from build123d import *

# Parameters (mm, degrees)
F0_W     = 676.275
F0_H     = 650.875
F1_DEPTH = 927.1
F3_DEPTH = 676.275
F4_W     = 473.075
F4_H     = 25.4
F5_DEPTH = 381


with BuildPart() as f1:
    # F0 (on Top) → F1 (new body)
    with BuildSketch(Plane.XY):
        with Locations((2.333625, 72.26744)):
            Rectangle(F0_W, F0_H)
    extrude(amount=F1_DEPTH)

    # F2 (on face) → F3 (join, through all)
    with BuildSketch(Plane(origin=(-335.803875, 0, 0), x_dir=(0, -1, 0), z_dir=(-1, 0, 0))):
        Polygon((-397.70494, 1104.9), (-397.70494, 927.1), (-269.652062, 927.1), (-372.30494, 1104.9), align=None)
    extrude(amount=-F3_DEPTH)

    # F4 (on face) → F5 (join)
    with BuildSketch(Plane.XY.offset(927.1)):
        with Locations((2.333625, 231.552062)):
            Rectangle(F4_W, F4_H)
    extrude(amount=F5_DEPTH)


solid = f1.part
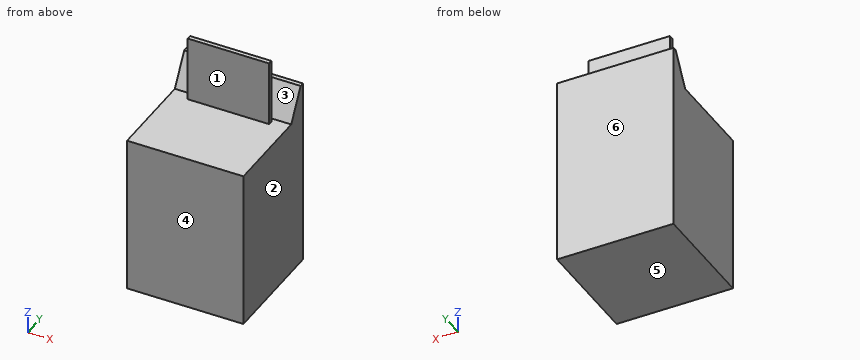
Input: part model. Units: mm. Frame: model coordinates. Face numbers are marked on the shaded views. A direction names the side the tool comes from. Coordinates: 2 decimals unless noted, no trailing zeros. Loops run counter-clockwise (first coordinate to the right, second up) from the corner with the lowest first, then second, coordinate; pieces in that order, holes last.
(1) Pull-direction query (Y, two-part tool) for the marked faces 3, 4, 5 and 6; classes: released by +Y, released by -Y, zero draft, split by the parting line, or undercut.
(2) Section A-A on x = -133.5. Return the cut outline in (y, z), then the cut area to 3 significant figures.
(3) Material intervals for probe 1 along Z at (x, y) = (278.5, 165); probe 2 along Y at (x, z) = (-85, 996); probe 3 along Y at (x, z) = (-88, 1067), sorted ascending.
(4) Section B-B on z = 1064.5. Return the cut outline in (x, y), then the cut area to 3 significant figures.
(5) Set-up query: the marked faces 1 and 2. Return all of +Z, -Z, +X, -X, +Y, -Y with unobstructed straight access to the full face (end or side cutting, diameter ignored); none if empty.
(6) First-contact query: pin 1 Ø12.5 at (x, y) = (163, 390) entering from +Z; pin 2 Ø12 at (x, z) = (209, 933.5) entering from -Y; pin 3 Ø7.5 at (y, z) = (225.5, 1161) entering from +X. Flat tips, straight axial feed; report the tip coordinate or a pass-through.
(7) Section C-C on y = -89. Return the cut outline in (x, z).
(8) Section D-D on x = 287. Return the cut outline in (y, z).
Data:
1. face 3: undercut
1. face 4: released by -Y
1. face 5: zero draft
1. face 6: released by +Y
2. outline: (-253.17, 0) - (397.7, 0) - (397.7, 1104.9) - (372.3, 1104.9) - (269.65, 927.1) - (244.25, 927.1) - (244.25, 1308.1) - (218.85, 1308.1) - (218.85, 927.1) - (-253.17, 927.1) - close
2. area: 627,000 mm2
3. probe 1: z = 0 to 927.1
3. probe 2: y = 218.85 to 244.25, 309.43 to 397.7
3. probe 3: y = 218.85 to 244.25, 350.42 to 397.7
4. outline: (-335.8, 348.98) - (340.47, 348.98) - (340.47, 397.7) - (-335.8, 397.7) - close; (-234.2, 218.85) - (238.87, 218.85) - (238.87, 244.25) - (-234.2, 244.25) - close
4. area: 45,000 mm2
5. face 1: +Z, +X, -X, -Y
5. face 2: +Z, -Z, +X, +Y, -Y
6. pin 1: stops at z = 1104.9
6. pin 2: stops at y = 218.85
6. pin 3: stops at x = 238.87
7. outline: (-335.8, 0) - (340.47, 0) - (340.47, 927.1) - (-335.8, 927.1) - close
8. outline: (-253.17, 0) - (397.7, 0) - (397.7, 1104.9) - (372.3, 1104.9) - (269.65, 927.1) - (-253.17, 927.1) - close
